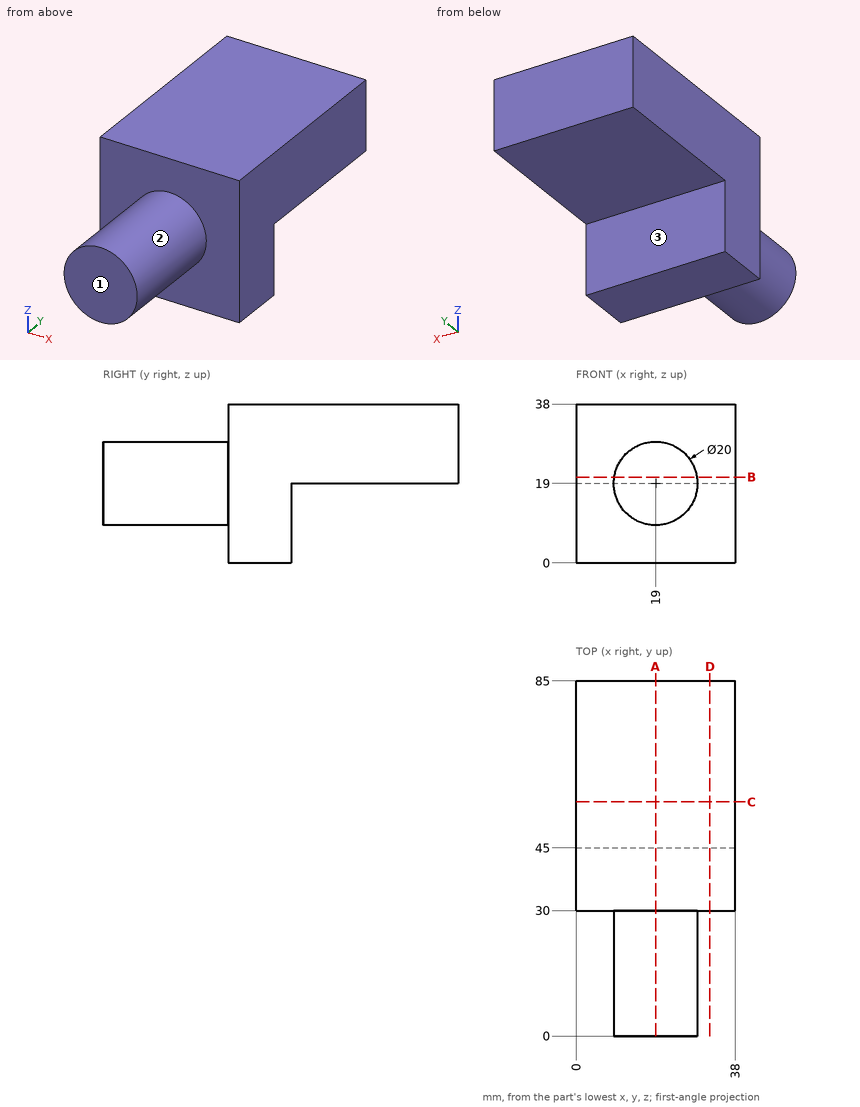
Source: three-view drawing plus pictorial views. Frame: mm from the lowest corner of the part. A direction names the side the tool comes from. Round coordinates to 2 decimals unless told otherwise and drop trailing zeros. Loops run counter-clockwise (first coordinate to the right, second up) from the corner with the lowest first, then second, coordinate; pieces in that order, holes last. Notation, with made-up numbers: (-40, 71) -> (5, 71) arc R32 cw to (5, 103) -> close; hole circle Ø11 at (79.5, 6). An arc over 180 degrees is marked (long way). Use one line per item in the form item = value.
Item 1: Cut plane C-C on y = 56. Output: boundary loops of the cut face in (x, z).
Evaluation:
outline = (0, 19) -> (38, 19) -> (38, 38) -> (0, 38) -> close
Item 2: Cut plane D-D on x = 32. Output: boundary loops of the cut face in (y, z).
Evaluation:
outline = (30, 0) -> (45, 0) -> (45, 19) -> (85, 19) -> (85, 38) -> (30, 38) -> close
Item 3: Access query for the marked faces 1, 2 and 3. Directions: +Z, -Z, +X, -X, +Y, -Y. A direction counts if a zero-diameter tool reaches every point of the face in a straight line with its end or side. Return the directions, or none.
Evaluation:
face_1 = +Z, -Z, +X, -X, -Y
face_2 = -Y
face_3 = -Z, +X, -X, +Y
Item 4: Cut plane A-A on x = 19. Output: boundary loops of the cut face in (y, z).
Evaluation:
outline = (0, 9) -> (30, 9) -> (30, 0) -> (45, 0) -> (45, 19) -> (85, 19) -> (85, 38) -> (30, 38) -> (30, 29) -> (0, 29) -> close
Item 5: Cut plane B-B on z = 20.5. Output: boundary loops of the cut face in (x, y).
Evaluation:
outline = (0, 30) -> (9.11, 30) -> (9.11, 0) -> (28.89, 0) -> (28.89, 30) -> (38, 30) -> (38, 85) -> (0, 85) -> close
Item 6: Contact query for flat-ended pins moving along their axis: pin 1 Ø19 at (x, z) = (11, 26.5) entering from -Y; pin 2 Ø6 at (x, z) = (22, 15.5) entering from +Y; pin 3 Ø19 at (x, y) = (28, 74.5) entering from -Z; pin 4 Ø1 at (x, z) = (29.5, 7.5) entering from -Y. Output: stop coordinate, or through.
Evaluation:
pin_1 = 0
pin_2 = 45
pin_3 = 19
pin_4 = 30
Item 7: Material intervals for probe 1 along Y at (x, z) = (7.5, 36); probe 2 along Y at (x, z) = (35, 8.5); probe 3 along Z at (x, y) = (22, 66.5), sorted ascending.
Evaluation:
probe_1 = 30 to 85
probe_2 = 30 to 45
probe_3 = 19 to 38
